```python
from build123d import *

# Parameters (mm, degrees)
SKETCH1_W                   = 6.35
SKETCH1_H                   = 12.7
BOSS_EXTRUDE1_DEPTH         = 398.018
F_34_0_111_DIAMETER_HOLE1_D = 2.8194
SKETCH6_W                   = 6.35
SKETCH6_H                   = 6.35
CUT_EXTRUDE1_DEPTH          = 7.35
TAP_DRILL_FOR_10_24_TAP1_D  = 3.7973
SKETCH9_W                   = 65.532
SKETCH9_H                   = 6.35
CUT_EXTRUDE3_DEPTH          = 7.35


with BuildPart() as part:
    # Sketch1 → Boss-Extrude1 (new body)
    with BuildSketch(Plane(origin=(0, 0, 0), x_dir=(0, 0, -1), z_dir=(1, 0, 0))):
        with Locations((3.175, 6.35)):
            Rectangle(SKETCH1_W, SKETCH1_H)
    extrude(amount=BOSS_EXTRUDE1_DEPTH)

    # #34 (0.111) Diameter Hole1 (through all)
    with Locations(Plane(origin=(0, 12.7, 0), x_dir=(1, 0, 0), z_dir=(0, 1, 0))):
        with Locations((3.175, 3.175), (159.131, 3.175), (80.899, 3.175), (237.363, 3.175), (315.595, 3.175), (394.843, 3.175)):
            Hole(F_34_0_111_DIAMETER_HOLE1_D / 2)

    # Sketch6 → Cut-Extrude1 (cut, through all)
    with BuildSketch(Plane.XY):
        with Locations((315.595, 12.7)):
            Rectangle(SKETCH6_W, SKETCH6_H)
        with Locations((159.131, 12.7)):
            Rectangle(SKETCH6_W, SKETCH6_H)
        with Locations((3.175, 12.7)):
            Rectangle(SKETCH6_W, SKETCH6_H)
    extrude(amount=-CUT_EXTRUDE1_DEPTH, mode=Mode.SUBTRACT)

    # Tap Drill for #10-24 Tap1 (through all)
    with Locations(Plane.XY):
        with Locations((388.493, 6.35)):
            Hole(TAP_DRILL_FOR_10_24_TAP1_D / 2)

    # Sketch9 → Cut-Extrude3 (cut, through all)
    with BuildSketch(Plane.XY):
        with Locations((201.422, 3.175)):
            Rectangle(SKETCH9_W, SKETCH9_H)
        with Locations((273.304, 3.175)):
            Rectangle(SKETCH9_W, SKETCH9_H)
    extrude(amount=-CUT_EXTRUDE3_DEPTH, mode=Mode.SUBTRACT)


solid = part.part
```
The model under review builds one solid part; all positions refer to its coordinate system, in mm. A direction names the side the tool comes from. Coordinates: 2 decimals unless noted, no trailing zeros. Write each loop counter-clockwise with the first axis right and the second up, starting at its lowest first coordinate (ties: lowest second). Pieces come first, ordered by that corner, then holes. Notation, with made-up numbers: (17, 13) - (40, 13) arc R18 cw to (40, 24) - close; hole circle Ø9 at (39, 49.25). An arc over 180 degrees is marked (long way). Answer in a Markdown table with one row per item. Add a question column.
Q1. Consider section A-A on x = 255. Give the boundary of the cut face in (y, z).
Q2. Clearance check with flat-ended pins moving along their axes: pin 1 (1 mm diameter, centred on x = 295, z = -2, fed in from -Y); pin 2 (1.9 mm diameter, centred on x = 3, z = -2, fed in from +Y) (3 decimals); pin 3 (3.5 mm diameter, centred on y = 11.5, z = -3, fed in from -X). State where each tip first meets the part, or that it passes through.
Q3. To check wall thickness, follow line 1 along X through (y, z) = (10, -3); line 2 along X through (y, z) = (11.5, -1.25); line 3 along X through (y, z) = (5, -1). State the ranges of each line that lie inside material, in increasing order. Write a range as from..to.
Q4. For faces 4 (the face through (240.538, 3, -3)), 5 (the face through (2, 9.525, -2)), 6 (the face through (314, 9.525, -3)), 7 (the face through (196, 8, -6.35)), list the 3-axis set-ups (+Z, -Z, +X, -X, +Y, -Y) from which the entire face can be reached by the end or side of a thin tool; tool diameter is ignored.
Q5. Draft analysis for pull direction X (two halves, no side actions). For faces 1 (the face through (0, 5, -3)), 2 (the face through (234.188, 3, -3)), 3 (the face through (351, 0, -3)), state which applies: +X half, -X half, draft (parallel to the pull), parting line (faces both ways), or undercut.
Answers below:
| question | item | result |
|---|---|---|
| 1 | outline | (6.35, -6.35) - (12.7, -6.35) - (12.7, 0) - (6.35, 0) - close |
| 2 | pin 1 | y = 6.35 |
| 2 | pin 2 | y = 9.525 |
| 2 | pin 3 | x = 6.35 |
| 3 | line 1 | 6.35..79.5, 82.3..155.96, 162.31..235.96, 238.76..312.42, 318.77..393.44, 396.24..398.02 |
| 3 | line 2 | 6.35..155.96, 162.31..312.42, 318.77..398.02 |
| 3 | line 3 | 0..168.66, 234.19..240.54, 306.07..387.16, 389.83..398.02 |
| 4 | face 4 | +Z, -Z, -Y |
| 4 | face 5 | +Z, -Z, -X, +Y |
| 4 | face 6 | +Z, -Z, +Y |
| 4 | face 7 | -Z, +X, -X, +Y, -Y |
| 5 | face 1 | -X half |
| 5 | face 2 | undercut |
| 5 | face 3 | draft |
